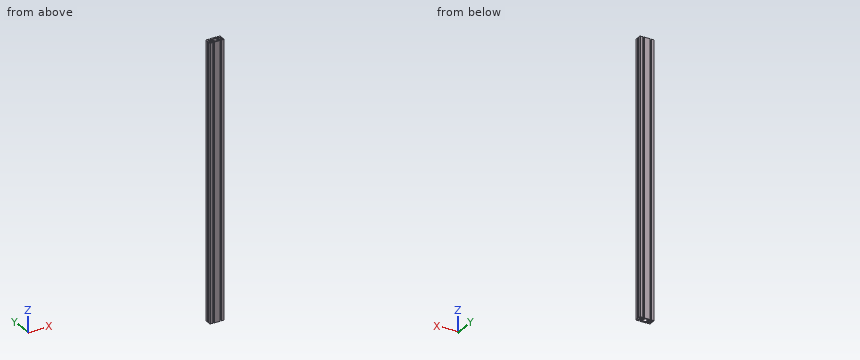
from build123d import *

# Parameters (mm, degrees)
SKETCH3_R           = 3.5
BOSS_EXTRUDE1_DEPTH = 762


with BuildPart() as part:
    # Sketch3 → Boss-Extrude1 (new, symmetric)
    with BuildSketch(Plane.XY):
        with BuildLine():
            Line((15.25, 20), (-15.25, 20))
            ThreePointArc((-15.25, 20), (-15.780330086, 19.780330086), (-16, 19.25))
            Line((-16, 19.25), (-16, 16.25))
            ThreePointArc((-16, 16.25), (-15.780330086, 15.719669914), (-15.25, 15.5))
            Line((-15.25, 15.5), (-9.931980515, 15.5))
            ThreePointArc((-9.931980515, 15.5), (-9.070942793, 14.924672987), (-9.272970773, 13.909009742))
            Line((-9.272970773, 13.909009742), (-15.140128061, 8.041852455))
            ThreePointArc((-15.140128061, 8.041852455), (-15.740311256, 7.640822865), (-16.448275606, 7.5))
            Line((-16.448275606, 7.5), (-23.551724394, 7.5))
            ThreePointArc((-23.551724394, 7.5), (-24.259688744, 7.640822865), (-24.859871939, 8.041852455))
            Line((-24.859871939, 8.041852455), (-30.727029227, 13.909009742))
            ThreePointArc((-30.727029227, 13.909009742), (-30.929057207, 14.924672987), (-30.068019485, 15.5))
            Line((-30.068019485, 15.5), (-24.75, 15.5))
            ThreePointArc((-24.75, 15.5), (-24.219669914, 15.719669914), (-24, 16.25))
            Line((-24, 16.25), (-24, 19.25))
            ThreePointArc((-24, 19.25), (-24.219669914, 19.780330086), (-24.75, 20))
            Line((-24.75, 20), (-37, 20))
            ThreePointArc((-37, 20), (-39.121320344, 19.121320344), (-40, 17))
            Line((-40, 17), (-40, 4.75))
            ThreePointArc((-40, 4.75), (-39.780330086, 4.219669914), (-39.25, 4))
            Line((-39.25, 4), (-36.25, 4))
            ThreePointArc((-36.25, 4), (-35.719669914, 4.219669914), (-35.5, 4.75))
            Line((-35.5, 4.75), (-35.5, 10.068019485))
            ThreePointArc((-35.5, 10.068019485), (-34.924672987, 10.929057207), (-33.909009742, 10.727029227))
            Line((-33.909009742, 10.727029227), (-28.041852455, 4.859871939))
            ThreePointArc((-28.041852455, 4.859871939), (-27.640822865, 4.259688744), (-27.5, 3.551724394))
            Line((-27.5, 3.551724394), (-27.5, -3.551724394))
            ThreePointArc((-27.5, -3.551724394), (-27.640822865, -4.259688744), (-28.041852455, -4.859871939))
            Line((-28.041852455, -4.859871939), (-33.909009742, -10.727029227))
            ThreePointArc((-33.909009742, -10.727029227), (-34.924672987, -10.929057207), (-35.5, -10.068019485))
            Line((-35.5, -10.068019485), (-35.5, -4.75))
            ThreePointArc((-35.5, -4.75), (-35.719669914, -4.219669914), (-36.25, -4))
            Line((-36.25, -4), (-39.25, -4))
            ThreePointArc((-39.25, -4), (-39.780330086, -4.219669914), (-40, -4.75))
            Line((-40, -4.75), (-40, -17))
            ThreePointArc((-40, -17), (-39.121320344, -19.121320344), (-37, -20))
            Line((-37, -20), (-24.75, -20))
            ThreePointArc((-24.75, -20), (-24.219669914, -19.780330086), (-24, -19.25))
            Line((-24, -19.25), (-24, -16.25))
            ThreePointArc((-24, -16.25), (-24.219669914, -15.719669914), (-24.75, -15.5))
            Line((-24.75, -15.5), (-30.068019485, -15.5))
            ThreePointArc((-30.068019485, -15.5), (-30.929057207, -14.924672987), (-30.727029227, -13.909009742))
            Line((-30.727029227, -13.909009742), (-24.859871939, -8.041852455))
            ThreePointArc((-24.859871939, -8.041852455), (-24.259688744, -7.640822865), (-23.551724394, -7.5))
            Line((-23.551724394, -7.5), (-16.448275606, -7.5))
            ThreePointArc((-16.448275606, -7.5), (-15.740311256, -7.640822865), (-15.140128061, -8.041852455))
            Line((-15.140128061, -8.041852455), (-9.272970773, -13.909009742))
            ThreePointArc((-9.272970773, -13.909009742), (-9.070942793, -14.924672987), (-9.931980515, -15.5))
            Line((-9.931980515, -15.5), (-15.25, -15.5))
            ThreePointArc((-15.25, -15.5), (-15.780330086, -15.719669914), (-16, -16.25))
            Line((-16, -16.25), (-16, -19.25))
            ThreePointArc((-16, -19.25), (-15.780330086, -19.780330086), (-15.25, -20))
            Line((-15.25, -20), (15.25, -20))
            ThreePointArc((15.25, -20), (15.780330086, -19.780330086), (16, -19.25))
            Line((16, -19.25), (16, -16.25))
            ThreePointArc((16, -16.25), (15.780330086, -15.719669914), (15.25, -15.5))
            Line((15.25, -15.5), (9.931980515, -15.5))
            ThreePointArc((9.931980515, -15.5), (9.070942793, -14.924672987), (9.272970773, -13.909009742))
            Line((9.272970773, -13.909009742), (15.140128061, -8.041852455))
            ThreePointArc((15.140128061, -8.041852455), (15.740311256, -7.640822865), (16.448275606, -7.5))
            Line((16.448275606, -7.5), (23.551724394, -7.5))
            ThreePointArc((23.551724394, -7.5), (24.259688744, -7.640822865), (24.859871939, -8.041852455))
            Line((24.859871939, -8.041852455), (30.727029227, -13.909009742))
            ThreePointArc((30.727029227, -13.909009742), (30.929057207, -14.924672987), (30.068019485, -15.5))
            Line((30.068019485, -15.5), (24.75, -15.5))
            ThreePointArc((24.75, -15.5), (24.219669914, -15.719669914), (24, -16.25))
            Line((24, -16.25), (24, -19.25))
            ThreePointArc((24, -19.25), (24.219669914, -19.780330086), (24.75, -20))
            Line((24.75, -20), (37, -20))
            ThreePointArc((37, -20), (39.121320344, -19.121320344), (40, -17))
            Line((40, -17), (40, -4.75))
            ThreePointArc((40, -4.75), (39.780330086, -4.219669914), (39.25, -4))
            Line((39.25, -4), (36.25, -4))
            ThreePointArc((36.25, -4), (35.719669914, -4.219669914), (35.5, -4.75))
            Line((35.5, -4.75), (35.5, -10.068019485))
            ThreePointArc((35.5, -10.068019485), (34.924672987, -10.929057207), (33.909009742, -10.727029227))
            Line((33.909009742, -10.727029227), (28.041852455, -4.859871939))
            ThreePointArc((28.041852455, -4.859871939), (27.640822865, -4.259688744), (27.5, -3.551724394))
            Line((27.5, -3.551724394), (27.5, 3.551724394))
            ThreePointArc((27.5, 3.551724394), (27.640822865, 4.259688744), (28.041852455, 4.859871939))
            Line((28.041852455, 4.859871939), (33.909009742, 10.727029227))
            ThreePointArc((33.909009742, 10.727029227), (34.924672987, 10.929057207), (35.5, 10.068019485))
            Line((35.5, 10.068019485), (35.5, 4.75))
            ThreePointArc((35.5, 4.75), (35.719669914, 4.219669914), (36.25, 4))
            Line((36.25, 4), (39.25, 4))
            ThreePointArc((39.25, 4), (39.780330086, 4.219669914), (40, 4.75))
            Line((40, 4.75), (40, 17))
            ThreePointArc((40, 17), (39.121320344, 19.121320344), (37, 20))
            Line((37, 20), (24.75, 20))
            ThreePointArc((24.75, 20), (24.219669914, 19.780330086), (24, 19.25))
            Line((24, 19.25), (24, 16.25))
            ThreePointArc((24, 16.25), (24.219669914, 15.719669914), (24.75, 15.5))
            Line((24.75, 15.5), (30.068019485, 15.5))
            ThreePointArc((30.068019485, 15.5), (30.929057207, 14.924672987), (30.727029227, 13.909009742))
            Line((30.727029227, 13.909009742), (24.859871939, 8.041852455))
            ThreePointArc((24.859871939, 8.041852455), (24.259688744, 7.640822865), (23.551724394, 7.5))
            Line((23.551724394, 7.5), (16.448275606, 7.5))
            ThreePointArc((16.448275606, 7.5), (15.740311256, 7.640822865), (15.140128061, 8.041852455))
            Line((15.140128061, 8.041852455), (9.272970773, 13.909009742))
            ThreePointArc((9.272970773, 13.909009742), (9.070942793, 14.924672987), (9.931980515, 15.5))
            Line((9.931980515, 15.5), (15.25, 15.5))
            ThreePointArc((15.25, 15.5), (15.780330086, 15.719669914), (16, 16.25))
            Line((16, 16.25), (16, 19.25))
            ThreePointArc((16, 19.25), (15.780330086, 19.780330086), (15.25, 20))
        make_face()
        with Locations((-20, 0)):
            Circle(SKETCH3_R, mode=Mode.SUBTRACT)
        with Locations(Location((20, 0, 0), (0, 0, 180))):
            Circle(SKETCH3_R, mode=Mode.SUBTRACT)
        with BuildLine():
            Line((-2.25, -14.568019485), (-11.958147545, -4.859871939))
            ThreePointArc((-11.958147545, -4.859871939), (-12.359177135, -4.259688744), (-12.5, -3.551724394))
            Line((-12.5, -3.551724394), (-12.5, 3.551724394))
            ThreePointArc((-12.5, 3.551724394), (-12.359177135, 4.259688744), (-11.958147545, 4.859871939))
            Line((-11.958147545, 4.859871939), (-2.25, 14.568019485))
            ThreePointArc((-2.25, 14.568019485), (0, 15.5), (2.25, 14.568019485))
            Line((2.25, 14.568019485), (11.958147545, 4.859871939))
            ThreePointArc((11.958147545, 4.859871939), (12.359177135, 4.259688744), (12.5, 3.551724394))
            Line((12.5, 3.551724394), (12.5, -3.551724394))
            ThreePointArc((12.5, -3.551724394), (12.359177135, -4.259688744), (11.958147545, -4.859871939))
            Line((11.958147545, -4.859871939), (2.25, -14.568019485))
            ThreePointArc((2.25, -14.568019485), (0, -15.5), (-2.25, -14.568019485))
        make_face(mode=Mode.SUBTRACT)
    extrude(amount=BOSS_EXTRUDE1_DEPTH, both=True)


solid = part.part
Work out the finished part from the listing and answer in its coordinate system (mm). Round coordinates to 2 decimals unless told otherwise and drop trailing zeros. Answer as CSV lines item,"result". Start each with the question number.
(1) The part is cut by section A-A, the plane z = 491. Give the number of separate pieces and of enclosed holes in the cut face, then the cut area to 3 significant figures.
(2) Find the intervals of material crossed by probe 1 along Y at (x, z) = (-26.5, 447); probe 2 along Y at (x, z) = (-15.5, 95); probe 3 along X at (y, z) = (-0.5, -395), in increasing order.
(3) Each of these flat-tipped pins is pushed along its axis until it touches: pin 1 (2.5 mm diameter, centred on y = 18, z = 176, fed in from +X); pin 2 (1.5 mm diameter, centred on x = -38, z = -18.5, fed in from +Y); pin 3 (2 mm diameter, centred on y = 0, z = 98.5, fed in from -X); pin 4 (2 mm diameter, centred on y = -1.5, z = 317.5, fed in from +X). Where does it stop, or does it pass through?
Output values:
1,separate pieces,"1"
1,enclosed holes,"3"
1,area,"1,590 mm²"
2,probe 1,"y = -20 to -15.5, -9.68 to 9.68, 15.5 to 20"
2,probe 2,"y = -19.96 to -15.54, -7.76 to 7.76, 15.54 to 19.96"
2,probe 3,"x = -27.5 to -23.46, -16.54 to -12.5, 12.5 to 16.54, 23.46 to 27.5"
3,pin 1,"stops at x = 40"
3,pin 2,"stops at y = 19.99"
3,pin 3,"stops at x = -27.5"
3,pin 4,"stops at x = 27.5"
